Read the model definition and answer for the solid it produces. Units are mm, in the model's axes. A direction names the side the tool comes from. Coordinates: 2 decimals unless noted, no trailing zeros. Loops run counter-clockwise (first coordinate to the right, second up) from the corner with the lowest first, then second, coordinate; pieces in that order, holes last. Notation, with made-up numbers: (59, 41.5) -> (111, 41.5) arc R9 cw to (111, 50.5) -> close; hole circle Ø10 at (76.5, 48.5). An arc over 180 degrees is marked (long way). Answer as a JSON object with one key per item and string values. Group by question number.
Q1. The part is cut by section C-C on x = 26.48. Write down the section's boundary in (y, z) (3 decimals).
Q2. Each of these flat-tipped pins is pushed along its axis until it touches: P1, Ø4.5, axis at x = 32.78, z = -19.755, coming from the -Y side; P2, Ø5, axis at x = 47.5, y = 28.5, coming from the -Z side. Where does it stop, or does it pass through?
Q3. The part is cut by section B-B on z = -33. Write down the section's boundary in (x, y).
Q4. Determine the mould class of faces 1 (the flat face through (20, 52, 2)), 2 (the flat face through (66.13, 50, -18)), 3 (the cylindrical face through (20.584, -21.394, -19.529)) for opening direction X: released by +X, released by -X, zero draft, split by the parting line, or undercut.
Q5. The part is cut by section A-A on x = -11. Write down the section's boundary in (y, z).
Q6. Straight lines are drawn through the part: line 1 along Y through (x, z) = (55, -29); line 2 along Z through (x, y) = (32.78, -21.3) (3 decimals); line 3 along X through (y, z) = (72.5, -27). For each, find the intervals that lie inside material, in ascending order. Write a range as [from, to].
Q7. The part is cut by section D-D on y = 14. Write down the section's boundary in (x, z), and give its area (3 significant figures).
Q8. For faces 4 (the cylindrical face through (35.28, -21.39, -19.82)), 5 (the flat face through (-25.29, 50, -18)), 6 (the flat face through (64.13, 50, -19)), determine the directions among +Z, -Z, +X, -X, +Y, -Y from which every point of the face is accessible in a straight line to the end or side of a thin tool.
from build123d import *

# Parameters (mm, degrees)
SKETCH_1_W          = 87.41993269
SKETCH_1_H          = 142.13
EXTRUDE_1_DEPTH     = 2
SKETCH_3_W          = 91.41993269
SKETCH_3_H          = 146.13
SKETCH_3_W_2        = 87.41993269
SKETCH_3_H_2        = 142.13
EXTRUDE_2_DEPTH     = 40.1
CUT_EXTRUDE_1_REACH = 166.86
SKETCH_4_W          = 27.46
SKETCH_4_H          = 8.31
SKETCH_4_W_2        = 17.9
SKETCH_4_H_2        = 4


with BuildPart() as part:
    # 草图1 → 凸台-拉伸1 (new body)
    with BuildSketch(Plane.XY):
        with Locations((20.419966345, 50.685)):
            Rectangle(SKETCH_1_W, SKETCH_1_H)
    extrude(amount=EXTRUDE_1_DEPTH)

    # 草图3 → 凸台-拉伸2 (add)
    with BuildSketch(Plane.XY.offset(2)):
        with Locations((20.419966345, 50.685)):
            Rectangle(SKETCH_3_W, SKETCH_3_H)
        with Locations((20.419966345, 50.685)):
            Rectangle(SKETCH_3_W_2, SKETCH_3_H_2, mode=Mode.SUBTRACT)
    extrude(amount=-EXTRUDE_2_DEPTH)

    # 草图4 → 切除-拉伸1 (cut, up to next)
    with BuildSketch(Plane.XZ.offset(22.38), mode=Mode.PRIVATE) as cut_extrude_1_sk1:
        with Locations((0, -19.755)):
            Rectangle(SKETCH_4_W, SKETCH_4_H)
    cut_extrude_1_tool1 = extrude(cut_extrude_1_sk1.sketch, amount=-CUT_EXTRUDE_1_REACH, mode=Mode.PRIVATE) & part.part
    # 草图4 → 切除-拉伸1 (cut, up to next)
    with BuildSketch(Plane.XZ.offset(22.38), mode=Mode.PRIVATE) as cut_extrude_1_sk2:
        with Locations((-7, -2)):
            Rectangle(SKETCH_4_W_2, SKETCH_4_H_2)
    cut_extrude_1_tool2 = extrude(cut_extrude_1_sk2.sketch, amount=-CUT_EXTRUDE_1_REACH, mode=Mode.PRIVATE) & part.part
    # 草图4 → 切除-拉伸1 (cut, up to next)
    with BuildSketch(Plane.XZ.offset(22.38), mode=Mode.PRIVATE) as cut_extrude_1_sk3:
        with BuildLine():
            ThreePointArc((31.896666667, -17.416256273), (20.58, -19.755), (31.896666667, -22.093743727))
            ThreePointArc((31.896666667, -22.093743727), (35.28, -19.755), (31.896666667, -17.416256273))
        make_face()
    cut_extrude_1_tool3 = extrude(cut_extrude_1_sk3.sketch, amount=-CUT_EXTRUDE_1_REACH, mode=Mode.PRIVATE) & part.part
    add(cut_extrude_1_tool1.solids().sort_by_distance((0, -22.38, -19.755))[0], mode=Mode.SUBTRACT)
    add(cut_extrude_1_tool2.solids().sort_by_distance((-7, -22.38, -2))[0], mode=Mode.SUBTRACT)
    add(cut_extrude_1_tool3.solids().sort_by_distance((27.210327, -22.38, -19.755))[0], mode=Mode.SUBTRACT)


solid = part.part
Final values:
{
 "1": {"outline": "(-22.38, -38.1) -> (-20.38, -38.1) -> (-20.38, -25.655) -> (-22.38, -25.655) -> close; (-22.38, -13.855) -> (-20.38, -13.855) -> (-20.38, 0) -> (121.75, 0) -> (121.75, -38.1) -> (123.75, -38.1) -> (123.75, 2) -> (-22.38, 2) -> close"},
 "2": {"P1": "stops at y = 121.75", "P2": "stops at z = 0"},
 "3": {"outline": "(-25.29, -22.38) -> (66.13, -22.38) -> (66.13, 123.75) -> (-25.29, 123.75) -> close; hole (-23.29, -20.38) -> (64.13, -20.38) -> (64.13, 121.75) -> (-23.29, 121.75) -> close"},
 "4": {"face 1": "zero draft", "face 2": "released by +X", "face 3": "undercut"},
 "5": {"outline": "(-22.38, -38.1) -> (-20.38, -38.1) -> (-20.38, -23.91) -> (-22.38, -23.91) -> close; (-22.38, -15.6) -> (-20.38, -15.6) -> (-20.38, -4) -> (-22.38, -4) -> close; (-22.38, 0) -> (121.75, 0) -> (121.75, -38.1) -> (123.75, -38.1) -> (123.75, 2) -> (-22.38, 2) -> close"},
 "6": {"line 1": "y = [-22.38, -20.38], [121.75, 123.75]", "line 2": "z = [-38.1, -22.255], [-17.255, 2]", "line 3": "x = [-25.29, -23.29], [64.13, 66.13]"},
 "7": {"outline": "(-25.29, -38.1) -> (-23.29, -38.1) -> (-23.29, 0) -> (64.13, 0) -> (64.13, -38.1) -> (66.13, -38.1) -> (66.13, 2) -> (-25.29, 2) -> close", "area": "335 mm2"},
 "8": {"face 4": "-Y", "face 5": "+Z, -Z, -X, +Y, -Y", "face 6": "-Z"}
}
